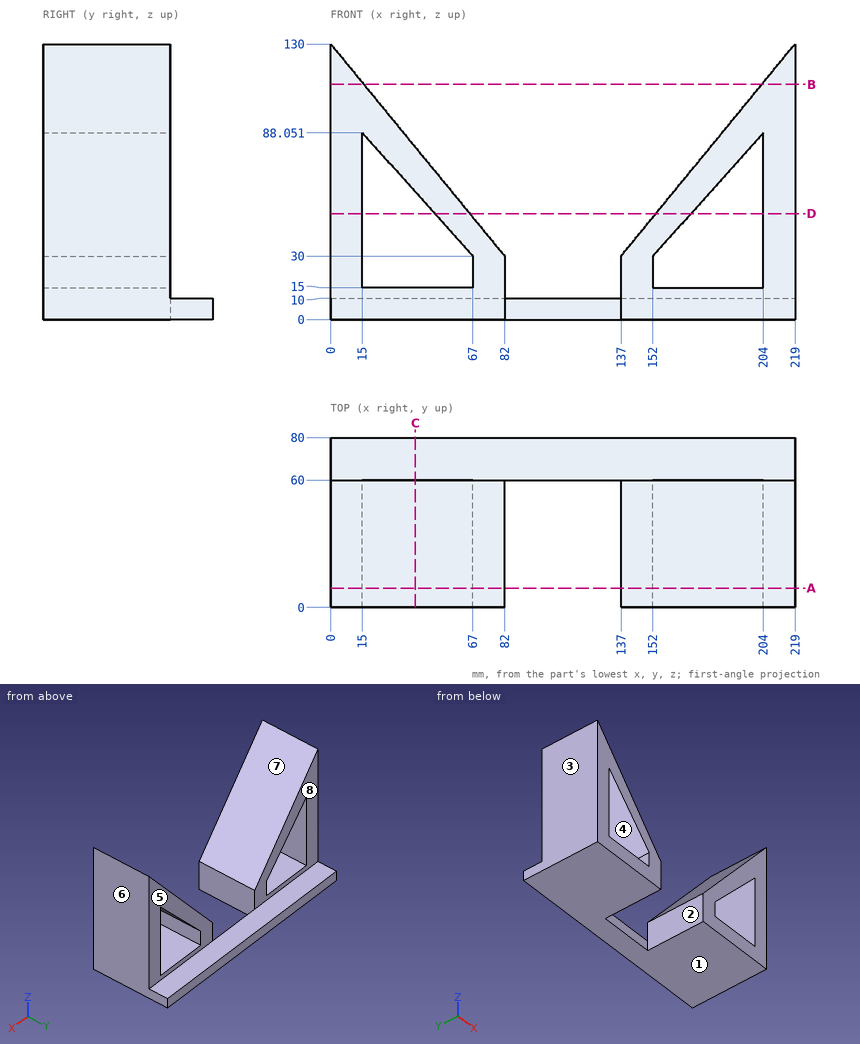
Here's the drawing with two shaded views (mm, measured from the low corner). I have some questions. A direction names the side the tool comes from. Coordinates: 2 decimals unless noted, no trailing zeros. Write each loop counter-clockwise with the first axis right and the second up, starting at its lowest first coordinate (ties: lowest second). Pieces come first, ordered by that corner, then holes. Notation, with made-up numbers: M 73,-28.5 L 90,-28.5 A24 cw 90,9.5 Z; hole C -35,-26.75 d6. An arc over 180 degrees is marked long. Answer as CSV lines item,"result". Start each with the question number.
1) I want a section at B-B, the plane z = 111. Please give me the cut outline in (x, y), and give its area (3 significant figures).
2) For the marked faces 1, 2, 3, 4 and 5, which set-ups out of +Z, -Z, +X, -X, +Y, -Y let a thin tool reach every point of the face, with its end or its side?
3) For P1, Ø8, axis at x = 176, y = 64.5, coming from the +Z side; P2, Ø5, axis at x = 46.5, y = 34.5, coming from the +Z side; P3, Ø3, axis at x = 123, z = 6, coming from the -Y side, each with a flat end and sliding along its axis, tell me the tip position at first contact or that it passes through.
4) I want a section at A-A, the plane y = 9. Please give me the cut outline in (x, z), and give its area (3 significant figures).
5) I want a section at D-D, the plane z = 50. Please give me the cut outline in (x, y), and give its area (3 significant figures).
6) We'd pull the mould along X, two halves only. Please class the marked faces 6, 7 and 8: +X half, -X half, draft (parallel to the pull), parting line (faces both ways), or undercut.
7) Please list where these lines run through material, in increasing order: line 1 (X direction, y = 12, z = 24.5); line 2 (X direction, y = 42.5, z = 69); line 3 (X direction, y = 53.5, z = 8). Write a range as from..to.
8) I want a section at C-C, the plane x = 40. Please give me the cut outline in (y, z), and give its area (3 significant figures).
Data:
1,outline,"M 0,0 L 15.58,0 L 15.58,60 L 0,60 Z; M 203.42,0 L 219,0 L 219,60 L 203.42,60 Z"
1,area,"1,870 mm^2"
2,face 1,"-Z, +X, -X, +Y, -Y"
2,face 2,"+Z, -Z, -Y"
2,face 3,"+Z, -Z, -X, +Y, -Y"
2,face 4,"+Y, -Y"
2,face 5,"+Z, +X, -X, +Y"
3,P1,"stops at z = 10"
3,P2,"stops at z = 76.34"
3,P3,"stops at y = 60"
4,outline,"M 0,0 L 82,0 L 82,30 L 0,130 Z; M 137,0 L 219,0 L 219,130 L 137,30 Z; hole M 15,15 L 67,15 L 67,30 L 15,88.05 Z; hole M 152,15 L 204,15 L 204,88.05 L 152,30 Z"
4,area,"8,540 mm^2"
5,outline,"M 0,0 L 15,0 L 15,60 L 0,60 Z; M 49.08,0 L 65.6,0 L 65.6,60 L 49.08,60 Z; M 153.4,0 L 169.92,0 L 169.92,60 L 153.4,60 Z; M 204,0 L 219,0 L 219,60 L 204,60 Z"
5,area,"3,780 mm^2"
6,face 6,"+X half"
6,face 7,"undercut"
6,face 8,"draft"
7,line 1,"x = 0..15, 67..82, 137..152, 204..219"
7,line 2,"x = 0..15, 32.07..50.02, 168.98..186.93, 204..219"
7,line 3,"x = 0..82, 137..219"
8,outline,"M 0,0 L 80,0 L 80,10 L 60,10 L 60,15 L 0,15 Z; M 0,60.14 L 60,60.14 L 60,81.22 L 0,81.22 Z"
8,area,"2,360 mm^2"
